For this review, take the finished solid that the model builds, in its own axes (mm). Face numbers are marked on the shaded views. Round coordinates to 2 decimals unless told otherwise and drop trailing zeros. Write each loop counter-clockwise with the first axis right and the second up, starting at its lowest first coordinate (ties: lowest second). Pieces come first, ordered by that corner, then holes. Notation, with made-up numbers: (61.5, 74.25) -> (92.5, 74.25) arc R25 ccw to (92.5, 99.25) -> close; hole circle Ø3 at (58.5, 10.25). An arc over 180 degrees is marked (long way). Answer in a Markdown table with one row per item.
from build123d import *

# Parameters (mm, degrees)
SKETCH1_R           = 82.5246
BOSS_EXTRUDE1_DEPTH = 38.1
SKETCH2_R           = 57.15
CUT_EXTRUDE1_DEPTH  = 38.1
SKETCH3_R           = 3.5687
CUT_EXTRUDE3_DEPTH  = 123.769007532
SKETCH4_R           = 5.5626
CUT_EXTRUDE4_DEPTH  = 9.652


with BuildPart() as part:
    # Sketch1 → Boss-Extrude1 (new body)
    with BuildSketch(Plane.YZ):
        with Locations(Location((0, 0, 0), (0, 0, 270))):
            Circle(SKETCH1_R)
    extrude(amount=BOSS_EXTRUDE1_DEPTH)

    # Sketch2 → Cut-Extrude1 (cut)
    with BuildSketch(Plane.YZ):
        with Locations(Location((0, 0, 0), (0, 0, 270))):
            Circle(SKETCH2_R)
    extrude(amount=CUT_EXTRUDE1_DEPTH, mode=Mode.SUBTRACT)

    # Sketch3 → Cut-Extrude3 (cut, through all)
    with BuildSketch(Plane.YZ):
        with Locations(Location((0, 73.025, 0), (0, 0, 270))):
            Circle(SKETCH3_R)
        with Locations(Location((-63.241505111, -36.5125, 0), (0, 0, 270))):
            Circle(SKETCH3_R)
        with Locations(Location((63.241505111, -36.5125, 0), (0, 0, 270))):
            Circle(SKETCH3_R)
    extrude(amount=CUT_EXTRUDE3_DEPTH, mode=Mode.SUBTRACT)

    # Sketch4 → Cut-Extrude4 (cut)
    with BuildSketch(Plane.YZ):
        with Locations(Location((0, 73.025, 0), (0, 0, 270))):
            Circle(SKETCH4_R)
        with Locations(Location((-63.241505111, -36.5125, 0), (0, 0, 270))):
            Circle(SKETCH4_R)
        with Locations(Location((63.241505111, -36.5125, 0), (0, 0, 270))):
            Circle(SKETCH4_R)
    extrude(amount=CUT_EXTRUDE4_DEPTH, mode=Mode.SUBTRACT)


solid = part.part
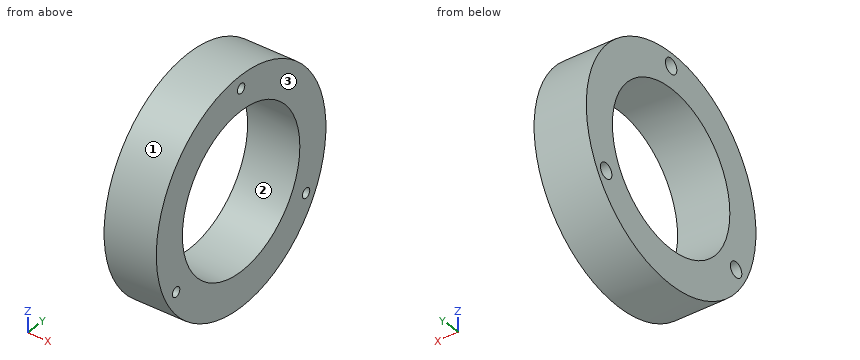
1) Consider section A-A on z = 0. State the section outline as (x, y) points, then the cut area to 3 significant figures.
Solved:
| item | result |
|---|---|
| outline | (0, -82.52) -> (38.1, -82.52) -> (38.1, -57.15) -> (0, -57.15) -> close; (0, 57.15) -> (38.1, 57.15) -> (38.1, 82.52) -> (0, 82.52) -> close |
| area | 1,930 mm² |
2) Consider section D-D on y = -19. State the section outline as (x, z) points.
Solved:
| item | result |
|---|---|
| outline | (0, -80.31) -> (38.1, -80.31) -> (38.1, -53.9) -> (0, -53.9) -> close; (0, 53.9) -> (38.1, 53.9) -> (38.1, 80.31) -> (0, 80.31) -> close |
3) Consider section C-C on x = 26.5. State how many separate pieces and enclosed holes the cut face has, then the cut area to 3 significant figures.
Solved:
| item | result |
|---|---|
| separate pieces | 1 |
| enclosed holes | 4 |
| area | 11,000 mm² |
4) For line 1 (Y direction, x = 19.5, z = -2) (3 decimals); line 2 (Y direction, x = 25.5, z = -14); line 3 (Z direction, x = 22, y = 2) (3 decimals), list the stretches that pass through material, from the lowest coordinate up. Write a range as [from, to].
Solved:
| item | result |
|---|---|
| line 1 | [-82.5, -57.115], [57.115, 82.5] |
| line 2 | [-81.33, -55.41], [55.41, 81.33] |
| line 3 | [-82.5, -57.115], [57.115, 70.069], [75.981, 82.5] |
5) Consider section B-B on y = 0. State the section outline as (x, z) points, then the cut area to 3 significant figures.
Solved:
| item | result |
|---|---|
| outline | (0, -82.52) -> (38.1, -82.52) -> (38.1, -57.15) -> (0, -57.15) -> close; (0, 57.15) -> (38.1, 57.15) -> (38.1, 69.46) -> (9.65, 69.46) -> (9.65, 67.46) -> (0, 67.46) -> close; (0, 78.59) -> (9.65, 78.59) -> (9.65, 76.59) -> (38.1, 76.59) -> (38.1, 82.52) -> (0, 82.52) -> close |
| area | 1,620 mm² |
6) Mouldability with a two-part tool opening along Z and no side actions: class the marked faces 1, 2 and 3 as pulls with the +Z half, pulls with the -Z half, needs draft (parallel to the pull), parting line crosses it, or undercut.
Solved:
| item | result |
|---|---|
| face 1 | parting line crosses it |
| face 2 | undercut |
| face 3 | needs draft |
7) Clearance check with flat-ended pins moving along their axes: pin 1 Ø6 at (x, y) = (13.5, -18) entering from -Z; pin 2 Ø4 at (x, y) = (17, -45) entering from +Z; pin 3 Ø12 at (x, z) = (20, 7.5) entering from -Y. State where each tip first meets the part, or that it passes through.
Solved:
| item | result |
|---|---|
| pin 1 | z = -81.15 |
| pin 2 | z = 70.44 |
| pin 3 | y = -82.51 |
